```python
from build123d import *

# Parameters (mm, degrees)
CHAMFER1_SIZE = 5
FILLET1_R     = 10
FILLET2_R     = 40
FILLET3_R     = 5


with BuildPart() as part:
    # Sketch25 → Revolve1 (revolve)
    with BuildSketch(Plane.XY, mode=Mode.PRIVATE) as revolve1_sk:
        Polygon((180, 60), (260, 60), (260, 421.608554244), (250, 431.608554244), (250, 457.288046169), (240, 494.608554244), (240, 544.608554244), (250, 544.608554244), (250, 669.608554244), (180, 669.608554244), align=None)
    revolve(revolve1_sk.sketch.rotate(Axis((180, 669.608554244, 0), (0, -1, 0)), 90), axis=Axis((180, 669.608554244, 0), (0, -1, 0)))

    # Chamfer1
    chamfer1_edges = [part.edges().sort_by_distance(p)[0] for p in [
        (180, 669.608554244, -70),
    ]]
    chamfer(chamfer1_edges, length=CHAMFER1_SIZE)

    # Fillet1
    fillet1_edges = [part.edges().sort_by_distance(p)[0] for p in [
        (180, 544.608554244, -60),
    ]]
    fillet(fillet1_edges, radius=FILLET1_R - 0.0001)  # a hair under: the kernel refuses the full size

    # Fillet2
    fillet2_edges = [part.edges().sort_by_distance(p)[0] for p in [
        (180, 494.608554244, -60),
        (180, 457.288046169, -70),
    ]]
    fillet(fillet2_edges, radius=FILLET2_R)

    # Fillet3
    fillet3_edges = [part.edges().sort_by_distance(p)[0] for p in [
        (180, 431.608554244, -70),
    ]]
    fillet(fillet3_edges, radius=FILLET3_R)


solid = part.part
```
Part model, mm, in its own coordinate system. A direction names the side the tool comes from. Coordinates: 2 decimals unless noted, no trailing zeros. Order: outer loops, then holes, each group sorted by start corner. A loop starts at its lowest first (then second) coordinate and runs counter-clockwise, first axis right, second up. Notation, with made-up numbers: (10.25, 52) - (60.25, 52) arc R14 ccw to (60.25, 62) - close; hole circle Ø5 at (35, -21.5). An arc over 180 degrees is marked (long way). Return JSON: item names as keys, results as strings. Group by question number.
Item 1: Which spindle directions (+Z, -Z, +X, -X, +Y, -Y) get a long thin tool onto all of the face, cutting with end or side? Do faces 5 (the face through (110.596, 605.449, -9.113)), 6 (the face through (179, 60, 1)). Say none if no direction does.
Item 2: Drill centre lines: probe 1 along Z at (x, y) = (181, 555.5); probe 2 along X at (y, z) = (101, 36); probe 3 along Z at (x, y) = (176, 388). Where is each one in solid material? Low to high. Write a range as from..to.
Item 3: Cut at B-B (y = 441). List the corners of the cut face in (x, z).
Item 4: Pin check, flat tips, straight feed: pin 1 (6 mm diameter, centred on x = 135, y = 604.5, fed in from +Z); pin 2 (2 mm diameter, centred on y = 367.5, z = -34, fed in from -X); pin 3 (1 mm diameter, centred on x = 118, y = 433.5, fed in from -Z). Stop position of each tip, or through.
Item 5: Pull direction Y, two halves, no side cores. Call faces 1 (the face through (179, 669.609, -1)), 2 (the face through (129.41, 517.48, 32.26)), 3 (the face through (100.68, 243.34, -10.41)), 4 (the face through (203.64, 488.2, 57.01)): pulls with the +Y half, pulls with the -Y half, needs draft (parallel to the pull), parting line crosses it, or undercut.
Item 6: Cut at A-A (y = 309). List the corners of the cut face in (x, z), plus the area to 3 significant figures.
Check values:
{
 "1": {"face 5": "+Y", "face 6": "+Z, -Z, +X, -X, -Y"},
 "2": {"probe 1": "z = -69.99..69.99", "probe 2": "x = 108.56..251.44", "probe 3": "z = -79.9..79.9"},
 "3": {"outline": "circle Ø140 at (180, 0)"},
 "4": {"pin 1": "stops at z = 56", "pin 2": "stops at x = 107.12", "pin 3": "stops at z = -33.44"},
 "5": {"face 1": "pulls with the +Y half", "face 2": "undercut", "face 3": "needs draft", "face 4": "undercut"},
 "6": {"outline": "circle Ø160 at (180, 0)", "area": "20,100 mm2"}
}
